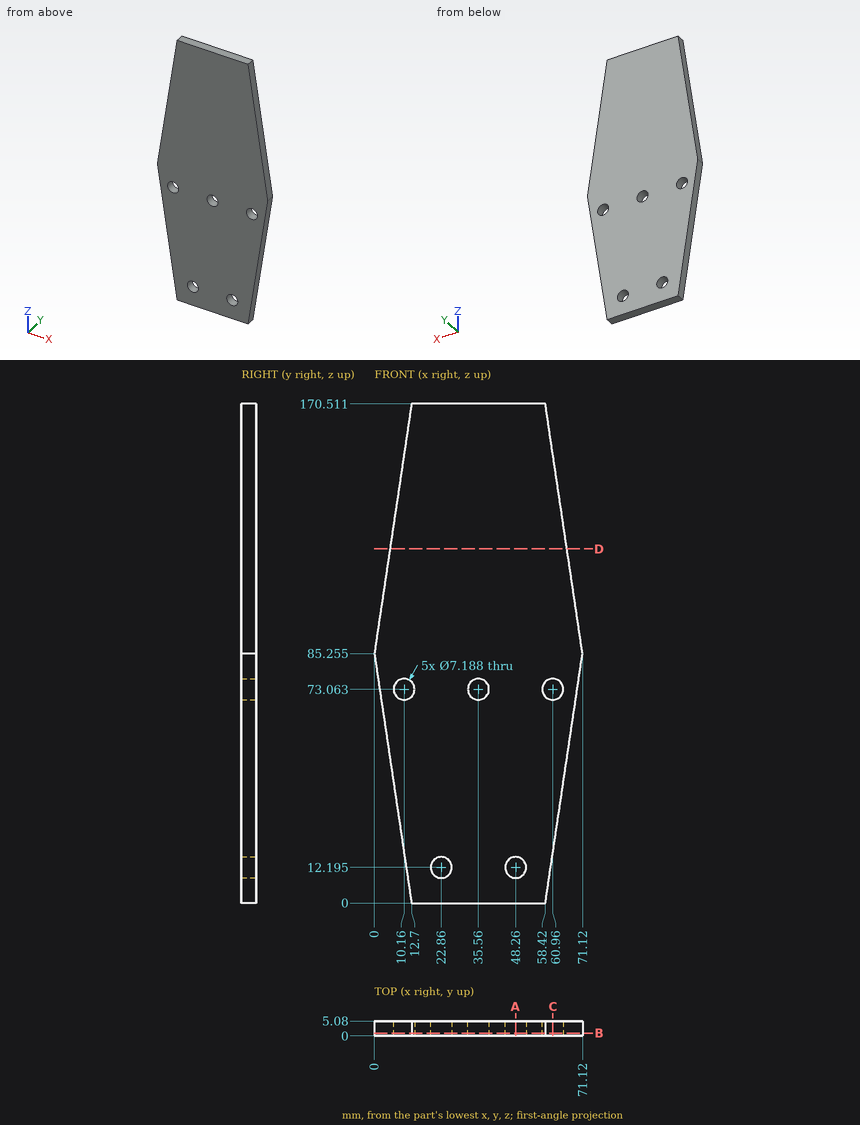
For this review, use the dimensioned drawing (mm, ordinates from the lowest corner) and the shaded views. Give positions to 0.01 mm unless a question says otherwise; leave off trailing zeros. Write each loop counter-clockwise with the first axis right and the second up, starting at its lowest first coordinate (ties: lowest second). Pieces come first, ordered by that corner, then holes. Notation, with made-up numbers: M 52,15.25 L 75,15.25 A11 ccw 75,29.25 Z; hole C -13.5,-32.5 d11. An arc over 180 degrees is marked long. Answer as a JSON object with one key per item and string values. Group by question number.
Item 1: Consider section B-B on y = 0.95. Write out the cut boundary in (x, z) (1 decimal), plus the area to 3 significant figures.
Item 2: For probe 1 along Z at (x, y) = (35.56, 3.8); probe 2 along X at (y, z) = (0.75, 9) (1 decimal); probe 3 along Z at (x, y) = (22.86, 1.9), list the stretches that pass through material, from the lowest coordinate up. Write a range as [from, to].
Item 3: Consider section C-C on x = 60.96. Write out the cut boundary in (y, z).
Item 4: Consider section A-A on x = 48.26. Write out the cut boundary in (y, z).
Item 5: Consider section D-D on z = 121. Write out the cut boundary in (x, y) (1 decimal), plus the area to 3 significant figures.
Check result:
{
 "1": {"outline": "M 0,85.3 L 12.7,0 L 58.4,0 L 71.1,85.3 L 58.4,170.5 L 12.7,170.5 Z; hole C 10.2,73.1 d7.2; hole C 22.9,12.2 d7.2; hole C 35.6,73.1 d7.2; hole C 48.3,12.2 d7.2; hole C 61,73.1 d7.2", "area": "9,760 mm^2"},
 "2": {"probe 1": "z = [0, 69.47], [76.66, 170.51]", "probe 2": "x = [11.4, 21.2], [24.5, 46.6], [49.9, 59.8]", "probe 3": "z = [0, 8.6], [15.79, 170.51]"},
 "3": {"outline": "M 0,17.05 L 5.08,17.05 L 5.08,69.47 L 0,69.47 Z; M 0,76.66 L 5.08,76.66 L 5.08,153.46 L 0,153.46 Z"},
 "4": {"outline": "M 0,0 L 5.08,0 L 5.08,8.6 L 0,8.6 Z; M 0,15.79 L 5.08,15.79 L 5.08,170.51 L 0,170.51 Z"},
 "5": {"outline": "M 5.3,0 L 65.8,0 L 65.8,5.1 L 5.3,5.1 Z", "area": "307 mm^2"}
}
